For this review, take the finished solid that the model builds, in its own axes (mm). A direction names the side the tool comes from. Round coordinates to 2 decimals unless told otherwise and drop trailing zeros. Loops run counter-clockwise (first coordinate to the right, second up) from the corner with the lowest first, then second, coordinate; pieces in that order, holes last.
1. Consider section A-A on y = 3.81. State the section outline as (x, z) points (3 decimals).
2. Tool access review of faces 1 (the flat face through (4, 1.65, 1)), 2 (the cylindrical face through (6.056, 11.615, -0.789)), 3 (the flat face through (3.6, 0, 1)), 4 (the flat face through (5.35, 0, 1)): name each direction out of +Z, -Z, +X, -X, +Y, -Y from which nothing blocks a thin tool from reaching the whole face with its end or side.
3. Clearance check with flat-ended pins moving along their axes: pin 1 Ø7.5 at (x, y) = (-3.5, 5) entering from +Z; pin 2 Ø0.5 at (x, z) = (4.5, 1) entering from -Y; pin 3 Ø5 at (x, y) = (5.25, 10.35) entering from -Z; pin 4 Ø1 at (y, z) = (0.5, 1) entering from +X. State where each tip first meets the part, or that it passes through.
4. Consider section B-B on z = -0.8. State how many separate pieces and enclosed holes the cut face has, then the cut area to 3 significant figures.
5. Consider section C-C on y = 10.35. State the section outline as (x, z) points.
6. Draft analysis for pull direction X (two halves, no side actions). For faces 5 (the flat face through (-7.65, 0, -1)), 6 (the cylindrical face through (-6.927, -4.099, -0.811)), 7 (the flat face through (7.65, 0, -1)), state which applies: released by +X, released by -X, zero draft, split by the parting line, or undercut.
7. To check wall thickness, follow line 1 along Y through (x, z) = (5.25, -0.6); line 2 along X through (y, z) = (11.5, -1.15); line 3 along X through (y, z) = (-0.25, 0.75). State the ranges of each line that lie inside material, in increasing order.
from build123d import *

# Parameters (mm, degrees)
SKETCH_1_W             = 15.3
SKETCH_1_H             = 26
EXTRUDE_1_DEPTH        = 1.6
CUT_EXTRUDE_1_REACH    = 17.168
SKETCH_2_R             = 1.5
SKETCH_3_W             = 1.75
SKETCH_3_H             = 3.3
EXTRUDE_2_DEPTH        = 1.9
CUT_EXTRUDE_2_REACH    = 17.203
SKETCH_4_R             = 0.475
PATTERN_LINEAR_1_COUNT = 5
PATTERN_LINEAR_1_PITCH = 2.54
MIRROR_START           = -1.6
MIRROR_1_OUTLINE_R     = 0.475
MIRROR_1_DEPTH         = 1.6


# Read off the part's stored shape, not the designer's step: the mirror step
with BuildPart() as part:
    # Sketch 1 → Extrude 1 (new body)
    with BuildSketch(Plane.XY):
        Rectangle(SKETCH_1_W, SKETCH_1_H)
    extrude(amount=-EXTRUDE_1_DEPTH)

    # Sketch 2 → Cut-Extrude 1 (cut, up to next)
    with BuildSketch(Plane.XY, mode=Mode.PRIVATE) as cut_extrude_1_sk1:
        with Locations((5.25, -10.35)):
            Circle(SKETCH_2_R)
    cut_extrude_1_tool1 = extrude(cut_extrude_1_sk1.sketch, amount=-CUT_EXTRUDE_1_REACH, mode=Mode.PRIVATE) & part.part
    # Sketch 2 → Cut-Extrude 1 (cut, up to next)
    with BuildSketch(Plane.XY, mode=Mode.PRIVATE) as cut_extrude_1_sk2:
        with Locations((5.25, 10.35)):
            Circle(SKETCH_2_R)
    cut_extrude_1_tool2 = extrude(cut_extrude_1_sk2.sketch, amount=-CUT_EXTRUDE_1_REACH, mode=Mode.PRIVATE) & part.part
    add(cut_extrude_1_tool1.solids().sort_by_distance((5.25, -10.35, 0))[0], mode=Mode.SUBTRACT)
    add(cut_extrude_1_tool2.solids().sort_by_distance((5.25, 10.35, 0))[0], mode=Mode.SUBTRACT)

    # Sketch 3 → Extrude 2 (add)
    with BuildSketch(Plane.XY):
        with Locations((4.475, 0)):
            Rectangle(SKETCH_3_W, SKETCH_3_H)
    extrude(amount=EXTRUDE_2_DEPTH)

    # Sketch 4 → Cut-Extrude 2 (cut, up to next)
    with BuildSketch(Plane.XY, mode=Mode.PRIVATE) as cut_extrude_2_sk1:
        with Locations((-6.55, 1.27)):
            Circle(SKETCH_4_R)
    cut_extrude_2_tool1 = extrude(cut_extrude_2_sk1.sketch, amount=-CUT_EXTRUDE_2_REACH, mode=Mode.PRIVATE) & part.part
    # Sketch 4 → Cut-Extrude 2 (cut, up to next)
    with BuildSketch(Plane.XY, mode=Mode.PRIVATE) as cut_extrude_2_sk2:
        with Locations((-6.55, -1.27)):
            Circle(SKETCH_4_R)
    cut_extrude_2_tool2 = extrude(cut_extrude_2_sk2.sketch, amount=-CUT_EXTRUDE_2_REACH, mode=Mode.PRIVATE) & part.part
    cut_extrude_2_1 = cut_extrude_2_tool1.solids().sort_by_distance((-6.55, 1.27, 0))[0]
    add(cut_extrude_2_1, mode=Mode.SUBTRACT)
    cut_extrude_2_2 = cut_extrude_2_tool2.solids().sort_by_distance((-6.55, -1.27, 0))[0]
    add(cut_extrude_2_2, mode=Mode.SUBTRACT)
    cut_extrude_2 = cut_extrude_2_1 + cut_extrude_2_2  # Cut-Extrude 2 as one shape, for the pattern or mirror that repeats it

    # Pattern Linear 1: Cut-Extrude 2 ×5
    with Locations(*[(0, i * PATTERN_LINEAR_1_PITCH, 0) for i in range(1, PATTERN_LINEAR_1_COUNT)]):
        add(cut_extrude_2, mode=Mode.SUBTRACT)

    # Mirror 1 outline → Mirror 1 (cut)
    with BuildSketch(Plane.XY.offset(MIRROR_START)):
        with Locations((-6.55, -6.35)):
            Circle(MIRROR_1_OUTLINE_R)
        with Locations((-6.55, -3.81)):
            Circle(MIRROR_1_OUTLINE_R)
        with Locations((-6.55, -11.43)):
            Circle(MIRROR_1_OUTLINE_R)
        with Locations((-6.55, -8.89)):
            Circle(MIRROR_1_OUTLINE_R)
    extrude(amount=MIRROR_1_DEPTH, mode=Mode.SUBTRACT)


solid = part.part
Resolved:
1. outline: (-7.65, -1.6) - (-7.025, -1.6) - (-7.025, 0) - (-7.65, 0) - close; (-6.075, -1.6) - (7.65, -1.6) - (7.65, 0) - (-6.075, 0) - close
2. face 1: +Z, +X, -X, +Y
2. face 2: +Z, -Z
2. face 3: +Z, -X, +Y, -Y
2. face 4: +Z, +X, +Y, -Y
3. pin 1: stops at z = 0
3. pin 2: stops at y = -1.65
3. pin 3: stops at z = -1.6
3. pin 4: stops at x = 5.35
4. separate pieces: 1
4. enclosed holes: 12
4. area: 377 mm2
5. outline: (-7.65, -1.6) - (3.75, -1.6) - (3.75, 0) - (-7.65, 0) - close; (6.75, -1.6) - (7.65, -1.6) - (7.65, 0) - (6.75, 0) - close
6. face 5: released by -X
6. face 6: undercut
6. face 7: released by +X
7. line 1: y = -13 to -11.85, -8.85 to 8.85, 11.85 to 13
7. line 2: x = -7.65 to -7.02, -6.08 to 4.29, 6.21 to 7.65
7. line 3: x = 3.6 to 5.35
